Verification items for the finished model (mm, model axes). A direction names the side the tool comes from. Round coordinates to 2 decimals unless told otherwise and drop trailing zeros. Order: outer loops, then holes, each group sorted by start corner. A loop starts at its lowest first (then second) coordinate and runs counter-clockwise, first axis right, second up.
```python
from build123d import *

# Parameters (mm, degrees)
F0_W     = 54.61
F0_H     = 101.6
F1_DEPTH = 4.064
F2_W     = 12.7
F2_H     = 3.175
F3_DEPTH = 12.7
F5_DEPTH = 25.4
F6_W     = 3.175
F6_H     = 3.175
F7_DEPTH = 12.7
F9_DEPTH = 25.4


with BuildPart() as f1:
    # F0 (on Top) → F1 (new body)
    with BuildSketch(Plane.XY):
        Rectangle(F0_W, F0_H)
    extrude(amount=F1_DEPTH)

    # F2 (on face) → F3 (join)
    with BuildSketch(Plane.XY.offset(4.064)):
        with Locations((0, 44.929545)):
            Rectangle(F2_W, F2_H)
    extrude(amount=F3_DEPTH)

    # F4 (on face) → F5 (cut)
    with BuildSketch(Plane(origin=(0, 46.517045, 0), x_dir=(-1, 0, 0), z_dir=(0, 1, 0))):
        Polygon((-6.35, 16.764), (0, 13.105086), (6.35, 16.764), align=None)
    extrude(amount=-F5_DEPTH, mode=Mode.SUBTRACT)

    # F6 (on face) → F7 (join)
    with BuildSketch(Plane.XY.offset(4.064)):
        with Locations((-25.7175, -49.2125)):
            Rectangle(F6_W, F6_H)
        with Locations((25.7175, -49.2125)):
            Rectangle(F6_W, F6_H)
    extrude(amount=F7_DEPTH)

    # F8 (on face) → F9 (cut)
    with BuildSketch(Plane.XZ.offset(50.8)):
        Polygon((-24.13, 16.764), (-27.305, 16.764), (-24.13, 15.9004), align=None)
        Polygon((24.13, 15.911566), (27.305, 16.764), (24.13, 16.764), align=None)
    extrude(amount=-F9_DEPTH, mode=Mode.SUBTRACT)


solid = f1.part
```
1) Sectioned sample at C-C on x = 8.5. Record the cut outline in (y, z), then the cut area to 3 significant figures.
2) Draft check along X on faces 6 (the flat face through (0, 46.517, 9)), 7 (the flat face through (-24.13, -49, 10)), 8 (the flat face through (-6.35, 45, 10)). Enter one of: released by +X, released by -X, zero draft, split by the parting line, or undercut.
3) Sectioned sample at A-A on z = 6.5. Record the cut outline in (x, y) (3 decimals), then the cut area to 3 significant figures.
4) Sectioned sample at B-B on y = -19. Record the cut outline in (x, z) (3 decimals).
5) Go/stop test with flat-tipped pins: pin 1 Ø2 at (x, z) = (1, 13) entering from +Y; pin 2 Ø5 at (y, z) = (-34.5, 7.5) entering from +X; pin 3 Ø1 at (x, y) = (-15, -17.5) entering from -Z; pin 4 Ø1 at (x, z) = (25, 13.5) entering from +Y (3 decimals). Record where each tip stops, or that it passes through.
6) Scan lines: probe 1 along Z at (x, y) = (2.5, 23.5); probe 2 along Y at (x, z) = (-2, 14). Record each from-to range of solid material in increasing order.
7) Tool access check on faces 1 (the flat face through (0, 50.8, 2)), 2 (the flat face through (6.35, 45, 10)), 3 (the flat face through (-26, -47.625, 10)), 4 (the flat face through (0, 43.342, 9)), 5 (the flat face through (24.13, -49, 10)). Record the directions out of +Z, -Z, +X, -X, +Y, -Y that give a thin tool (end or side, any length) a straight path to the whole face; none if there is none.
Returned:
1. outline: (-50.8, 0) - (50.8, 0) - (50.8, 4.06) - (-50.8, 4.06) - close
1. area: 413 mm2
2. face 6: zero draft
2. face 7: undercut
2. face 8: released by -X
3. outline: (-27.305, -50.8) - (-24.13, -50.8) - (-24.13, -47.625) - (-27.305, -47.625) - close; (-6.35, 43.342) - (6.35, 43.342) - (6.35, 46.517) - (-6.35, 46.517) - close; (24.13, -50.8) - (27.305, -50.8) - (27.305, -47.625) - (24.13, -47.625) - close
3. area: 60.5 mm2
4. outline: (-27.305, 0) - (27.305, 0) - (27.305, 4.064) - (-27.305, 4.064) - close
5. pin 1: stops at y = 46.52
5. pin 2: passes through
5. pin 3: stops at z = 0
5. pin 4: stops at y = -47.625
6. probe 1: z = 0 to 4.06
6. probe 2: y = 43.34 to 46.52
7. face 1: +Z, -Z, +X, -X, +Y
7. face 2: +Z, +X, +Y, -Y
7. face 3: +Z, +X, -X, +Y
7. face 4: +Z, +X, -X, -Y
7. face 5: +Z, +Y, -Y
